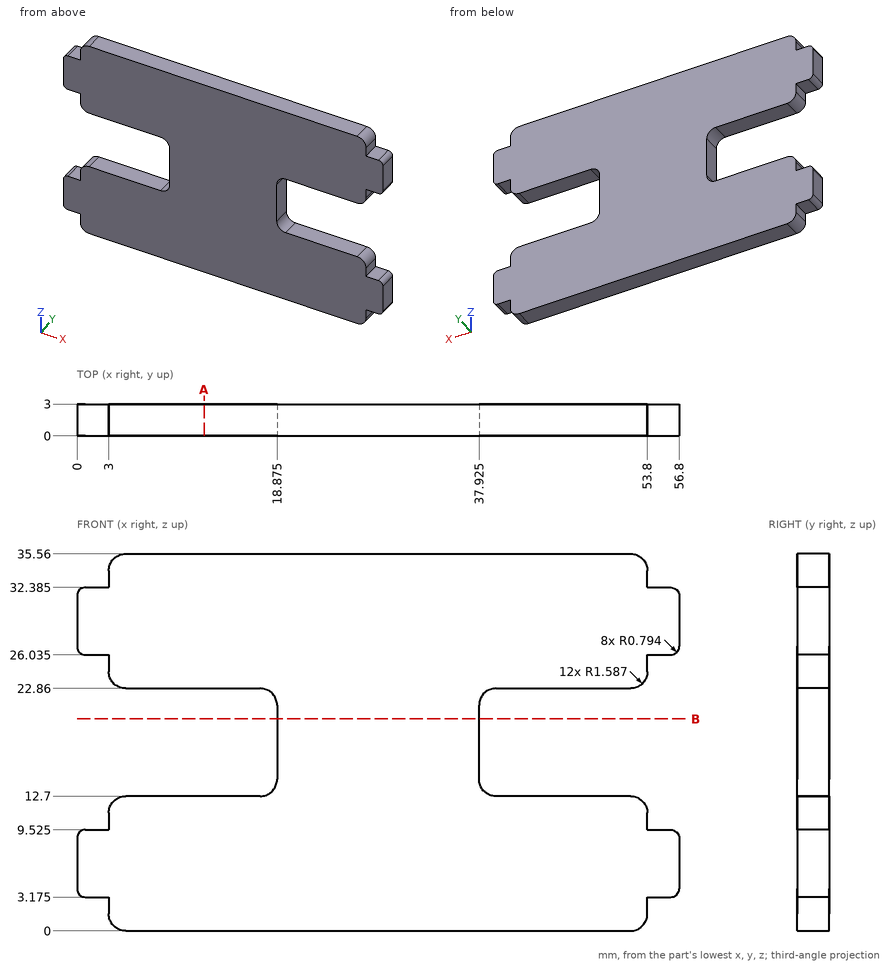
Verification items for this drawing (mm, ordinates from the low corner). Give positions to 0.01 mm unless a question says otherwise; leave off trailing zeros. Write each loop counter-clockwise with the first axis right and the second up, starting at its lowest first coordinate (ties: lowest second). Pieces come first, ordered by that corner, then holes. Notation, with made-up numbers: (14, 61) - (21, 61) arc R16 cw to (21, 76) - close; hole circle Ø3 at (82, 56.25). An arc over 180 degrees is marked (long way). Answer as a JSON object with one key per item and string values. Group by question number.
1) Sectioned sample at B-B (z = 20). Record the cut outline in (x, y) (1 decimal).
2) Sectioned sample at A-A (x = 12). Record the cut outline in (y, z).
3) Thickness scan on probe 1 along Z at (x, y) = (42.5, 0.8); probe 2 along X at (y, z) = (2, 24.5); probe 3 along X at (y, z) = (1.55, 17) (1 decimal). Record the ranges inside material, lowest first. Write a range as from..to.
4) Depth check by flat-ended pin: P1, Ø0.8, axis at y = 1, z = 25.5, coming from the +X side; P2, Ø0.7, axis at x = 55.5, y = 1, coming from the +Z side (1 decimal); P3, Ø0.8, axis at y = 1, z = 2.5, coming from the -X side. Enter the tip coordinate at first touch or a pass-through.
Geometry results:
{
 "1": {"outline": "(18.9, 0) - (37.9, 0) - (37.9, 3) - (18.9, 3) - close"},
 "2": {"outline": "(0, 0) - (3, 0) - (3, 12.7) - (0, 12.7) - close; (0, 22.86) - (3, 22.86) - (3, 35.56) - (0, 35.56) - close"},
 "3": {"probe 1": "z = 0..12.7, 22.86..35.56", "probe 2": "x = 3..53.8", "probe 3": "x = 18.9..37.9"},
 "4": {"P1": "stops at x = 53.8", "P2": "stops at z = 32.4", "P3": "stops at x = 3"}
}
